Geometry check sheet. Reference: the model listing, model coordinates, mm. Face numbers are marked on the shaded views. Give positions to 0.01 mm unless a question says otherwise; leave off trailing zeros. Loops run counter-clockwise (first coordinate to the right, second up) from the corner with the lowest first, then second, coordinate; pieces in that order, holes last. Notation, with made-up numbers: (-27.75, 35.5) - (12.25, 35.5) arc R34 cw to (12.25, 67.5) - close; hole circle Ø6 at (85.25, 38). An arc over 180 degrees is marked (long way). One line per question, with ' | ' between items. Start each with the question number.
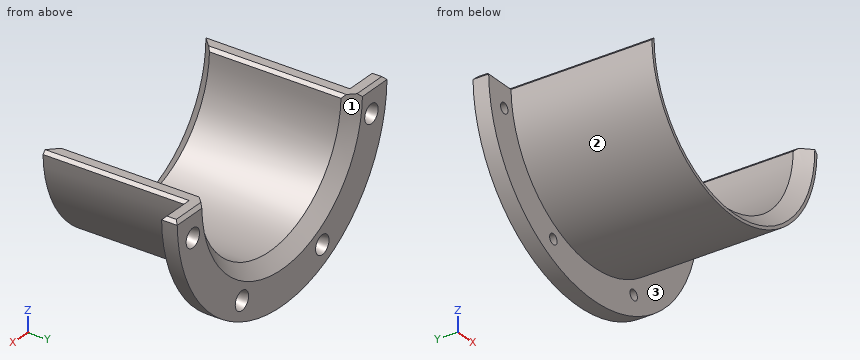
from build123d import *

# Parameters (mm, degrees)
PAD_DEPTH       = 50
PAD001_DEPTH    = 5
SKETCH003_R     = 3
POCKET_DEPTH    = 5
POCKET_TAPER    = 15
CHAMFER_SIZE    = 4
CHAMFER001_SIZE = 4
CHAMFER002_SIZE = 1


with BuildPart() as part:
    # Sketch → Pad (new body)
    with BuildSketch(Plane.XZ):
        with BuildLine():
            ThreePointArc((-37, 0), (0, -37), (37, 0))
            Line((32, 0), (37, 0))
            ThreePointArc((-32, 0), (0, -32), (32, 0))
            Line((-37, 0), (-32, 0))
        make_face()
    extrude(amount=PAD_DEPTH)

    # Sketch002 (on Face5 of Pad) → Pad001 (join)
    with BuildSketch(Plane(origin=(0, 0, 0), x_dir=(1, 0, 0), z_dir=(0, 1, 0))):
        with BuildLine():
            ThreePointArc((47, 0), (0, 47), (-47, 0))
            Line((-47, 0), (-37, 0))
            ThreePointArc((37, 0), (0, 37), (-37, 0))
            Line((37, 0), (47, 0))
        make_face()
    extrude(amount=-PAD001_DEPTH)

    # Sketch003 (on Face8 of Pad001) → Pocket (cut)
    with BuildSketch(Plane(origin=(0, 0, 0), x_dir=(1, 0, 0), z_dir=(0, 1, 0))):
        with Locations((-40, 8)):
            Circle(SKETCH003_R)
        with Locations((-18, 37)):
            Circle(SKETCH003_R)
        with Locations((18, 37)):
            Circle(SKETCH003_R)
        with Locations((40, 8)):
            Circle(SKETCH003_R)
    extrude(amount=-POCKET_DEPTH, taper=POCKET_TAPER, mode=Mode.SUBTRACT)

    # Chamfer
    chamfer_edges = [part.edges().sort_by_distance(p)[0] for p in [
        (0, -50, -32),
    ]]
    chamfer(chamfer_edges, length=CHAMFER_SIZE)

    # Chamfer001
    chamfer001_edges = [part.edges().sort_by_distance(p)[0] for p in [
        (0, 0, -32),
    ]]
    chamfer(chamfer001_edges, length=CHAMFER001_SIZE)

    # Chamfer002
    chamfer002_edges = [part.edges().sort_by_distance(p)[0] for p in [
        (-42, -5, 0),
        (-41.5, 0, 0),
        (-47, -2.5, 0),
        (-37, -27.5, 0),
        (-32, -25, 0),
        (42, -5, 0),
        (47, -2.5, 0),
        (41.5, 0, 0),
        (37, -27.5, 0),
        (32, -25, 0),
    ]]
    chamfer(chamfer002_edges, length=CHAMFER002_SIZE)


solid = part.part
(1) Depth check by flat-ended pin: pin 1 Ø3 at (y, z) = (-8, -35) entering from -X; pin 2 Ø10 at (y, z) = (-43, -19.5) entering from -X; pin 3 Ø3 at (y, z) = (-42, -26.5) entering from +X. Enter the tip coordinate at first touch or a pass-through.
(2) Mould release check, pull along X, two halves, no side actions. Record for the marked faces 1, 2 and 3: pulls with the +X half, pulls with the -X half, needs draft (parallel to the pull), parting line crosses it, or undercut.
(3) Section check D-D, the plane z = -43. Record the boundary of the cut face in (x, y).
(4) Material ranges on line 1 (Y direction, x = 32.5, z = -28); line 2 (X direction, y = -24, z = -16); line 3 (X direction, y = -7, z = -18), recorded low to high.
(5) Section check C-C, the plane z = -8. Count the separate pieces of the cut face and the enclosed holes in it, and give its area (3 significant figures).
(6) Section check B-B, the plane x = 40. Record the boundary of the cut face in (y, z), and give its area (3 significant figures).
Numbers:
1) pin 1: x = -15.71 | pin 2: x = -34.04 | pin 3: x = 27.28
2) face 1: undercut | face 2: parting line crosses it | face 3: needs draft
3) outline: (-18.97, -5) - (18.97, -5) - (18.97, 0) - (-18.97, 0) - close
4) line 1: -5 to 0 | line 2: -33.36 to -27.71, 27.71 to 33.36 | line 3: -32.33 to -26.46, 26.46 to 32.33
5) separate pieces: 4 | enclosed holes: 0 | area: 536 mm^2
6) outline: (-5, -24.68) - (0, -24.68) - (0, -11) - (-5, -9.66) - close; (-5, -6.34) - (0, -5) - (0, -1) - (-1, 0) - (-4, 0) - (-5, -1) - close | area: 99.1 mm^2
